Input: part model. Units: mm. Frame: model coordinates. Coordinates: 2 decimals unless noted, no trailing zeros. Write each loop counter-clockwise with the first axis right and the second up, starting at its lowest first coordinate (ties: lowest second). Pieces come first, ordered by that corner, then holes.
1) Draft query along Y for faces 1 (the flat face through (0, 8, 0)), 2 (the flat face through (-29, 47.6, 3)). Return one class per face: pulls with the +Y half, pulls with the -Y half, needs draft (parallel to the pull), parting line crosses it, or undercut.
2) Line query: L1, parallel to X at y = -28, z = 2 (3 decimals); L2, parallel to X at y = -68, z = 2; L3, parallel to X at y = 78, z = 5.5 (3 decimals). Output: solid intervals per line, ascending.
3) Section query D-D (y = -60.5). Output: boundary loops of the cut face in (x, z) (3 decimals).
4) Section query A-A (x = 24.5). State how many separate pieces and enclosed holes the cut face has, then the cut area to 3 significant figures.
5) Pin query (flat end, axial travel): pin 1 Ø3 at (x, z) = (24.5, 3.5) entering from +Y; pin 2 Ø8 at (x, y) = (-6, 2.5) entering from -Z. Return the tip coordinate at first contact, or that it passes through.
6) Section query C-C (y = 95.25). Output: boundary loops of the cut face in (x, z) (3 decimals).
7) Section query B-B (y = -95.25). Output: boundary loops of the cut face in (x, z) (3 decimals).
from build123d import *

# Parameters (mm, degrees)
F0_R     = 2.0701
F0_W     = 50.8
F0_H     = 27.6225
F1_DEPTH = 6.35


with BuildPart() as f1:
    # F0 (on Top) → F1 (new body)
    with BuildSketch(Plane.XY):
        Polygon((31.75, 76.2), (0, 76.2), (-31.75, 76.2), (-31.75, 101.6), (-57.15, 101.6), (-57.15, -101.6), (0, -101.6), (57.15, -101.6), (57.15, 101.6), (31.75, 101.6), align=None)
        with Locations((-50.8, -95.25)):
            Circle(F0_R, mode=Mode.SUBTRACT)
        with Locations((-50.8, -67.945)):
            Circle(F0_R, mode=Mode.SUBTRACT)
        Polygon((-3.175, -98.425), (-47.625, -98.425), (-47.625, -92.075), (-53.975, -92.075), (-53.975, -71.12), (-47.625, -71.12), (-3.175, -71.12), align=None, mode=Mode.SUBTRACT)
        Polygon((-47.625, -64.77), (-53.975, -64.77), (-53.975, -37.1475), (-3.175, -37.1475), (-3.175, -64.77), align=None, mode=Mode.SUBTRACT)
        with Locations((-28.575, -16.98625)):
            Rectangle(F0_W, F0_H, mode=Mode.SUBTRACT)
        Polygon((47.625, -71.12), (53.975, -71.12), (53.975, -92.075), (47.625, -92.075), (47.625, -98.425), (3.175, -98.425), (3.175, -71.12), align=None, mode=Mode.SUBTRACT)
        with Locations((50.8, -95.25)):
            Circle(F0_R, mode=Mode.SUBTRACT)
        Polygon((53.975, -37.1475), (53.975, -64.77), (47.625, -64.77), (3.175, -64.77), (3.175, -37.1475), align=None, mode=Mode.SUBTRACT)
        with Locations((50.8, -67.945)):
            Circle(F0_R, mode=Mode.SUBTRACT)
        with Locations((28.575, -16.98625)):
            Rectangle(F0_W, F0_H, mode=Mode.SUBTRACT)
        with Locations((-50.8, 25.3492)):
            Circle(F0_R, mode=Mode.SUBTRACT)
        Polygon((-53.975, 3.175), (-53.975, 22.1742), (-47.625, 22.1742), (-3.175, 22.1742), (-3.175, 3.175), align=None, mode=Mode.SUBTRACT)
        Polygon((-53.975, 28.5242), (-53.975, 47.5996), (-3.175, 47.5996), (-3.175, 28.5242), (-47.625, 28.5242), align=None, mode=Mode.SUBTRACT)
        with Locations((-50.8, 95.25)):
            Circle(F0_R, mode=Mode.SUBTRACT)
        Polygon((-34.925, 73.025), (-3.175, 73.025), (-3.175, 53.9496), (-53.975, 53.9496), (-53.975, 92.075), (-47.625, 92.075), (-47.625, 98.425), (-34.925, 98.425), align=None, mode=Mode.SUBTRACT)
        Polygon((53.975, 3.175), (3.175, 3.175), (3.175, 22.1742), (47.625, 22.1742), (53.975, 22.1742), align=None, mode=Mode.SUBTRACT)
        with Locations((50.8, 25.3492)):
            Circle(F0_R, mode=Mode.SUBTRACT)
        Polygon((3.175, 47.5996), (53.975, 47.5996), (53.975, 28.5242), (47.625, 28.5242), (3.175, 28.5242), align=None, mode=Mode.SUBTRACT)
        Polygon((3.175, 53.9496), (3.175, 73.025), (34.925, 73.025), (34.925, 98.425), (47.625, 98.425), (47.625, 92.075), (53.975, 92.075), (53.975, 53.9496), align=None, mode=Mode.SUBTRACT)
        with Locations((50.8, 95.25)):
            Circle(F0_R, mode=Mode.SUBTRACT)
    extrude(amount=F1_DEPTH)


solid = f1.part
Answer:
1. face 1: needs draft
1. face 2: undercut
2. L1: x = -57.15 to -53.975, -3.175 to 3.175, 53.975 to 57.15
2. L2: x = -57.15 to -52.87, -48.73 to 48.73, 52.87 to 57.15
2. L3: x = -57.15 to -53.975, -34.925 to -31.75, 31.75 to 34.925, 53.975 to 57.15
3. outline: (-57.15, 0) - (-53.975, 0) - (-53.975, 6.35) - (-57.15, 6.35) - close; (-3.175, 0) - (3.175, 0) - (3.175, 6.35) - (-3.175, 6.35) - close; (53.975, 0) - (57.15, 0) - (57.15, 6.35) - (53.975, 6.35) - close
4. separate pieces: 7
4. enclosed holes: 0
4. area: 242 mm2
5. pin 1: stops at y = 76.2
5. pin 2: stops at z = 0
6. outline: (-57.15, 0) - (-52.87, 0) - (-52.87, 6.35) - (-57.15, 6.35) - close; (-48.73, 0) - (-47.625, 0) - (-47.625, 6.35) - (-48.73, 6.35) - close; (-34.925, 0) - (-31.75, 0) - (-31.75, 6.35) - (-34.925, 6.35) - close; (31.75, 0) - (34.925, 0) - (34.925, 6.35) - (31.75, 6.35) - close; (47.625, 0) - (48.73, 0) - (48.73, 6.35) - (47.625, 6.35) - close; (52.87, 0) - (57.15, 0) - (57.15, 6.35) - (52.87, 6.35) - close
7. outline: (-57.15, 0) - (-52.87, 0) - (-52.87, 6.35) - (-57.15, 6.35) - close; (-48.73, 0) - (-47.625, 0) - (-47.625, 6.35) - (-48.73, 6.35) - close; (-3.175, 0) - (3.175, 0) - (3.175, 6.35) - (-3.175, 6.35) - close; (47.625, 0) - (48.73, 0) - (48.73, 6.35) - (47.625, 6.35) - close; (52.87, 0) - (57.15, 0) - (57.15, 6.35) - (52.87, 6.35) - close
